For this review, take the finished solid that the model builds, in its own axes (mm). Coordinates: 2 decimals unless noted, no trailing zeros. Write each loop counter-clockwise with the first axis right and the second up, starting at its lowest first coordinate (ties: lowest second). Pieces come first, ordered by that corner, then holes. Notation, with made-up numbers: M -9,68 L 6,68 A9 cw 6,72 Z; hole C 17.5,64.25 d4. An arc over 180 degrees is marked long. Return JSON: item names as keys, results as strings.
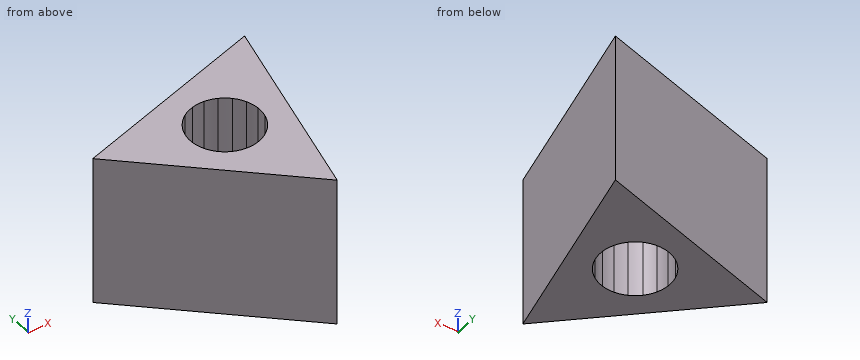
Autodesk Inventor part; units mm, degrees
ref_plane "Work Plane1" through (-2.6657, -0.4604, -13) normal (0, 0, -1) x (0, 1, 0)
ref_plane "YZ Plane" through (0, 0, 0) normal (1, 0, 0) x (0, 1, 0)
ref_plane "XZ Plane" through (0, 0, 0) normal (0, 1, 0) x (-1, 0, 0)
sketch "Sketch1" plane through (0, 0, 0) normal (0, 0, 1) x (1, 0, 0)
  line L0 (-1.6614, 3.5785) -> (-2.5268, 3.4417)
  line L1 (-2.0457, 4.3659) -> (-1.6614, 3.5785)
  line L2 (-1.1857, 4.1985) -> (-2.0457, 4.3659)
  line L3 (-1.2776, 5.0698) -> (-1.1857, 4.1985)
  line L4 (-0.5267, 4.6183) -> (-1.2776, 5.0698)
  line L5 (-0.315, 5.4685) -> (-0.5267, 4.6183)
  line L6 (-0.5267, 4.6183) -> (-0.315, 5.4685)
  arc A0 (-0.315, 5.4685) -> (-1.2776, 5.0698) centre (0.3343, 2.5396) ccw
  line L7 (-1.2776, 5.0698) -> (-0.5267, 4.6183)
  arc A1 (-1.2776, 5.0698) -> (-2.0457, 4.3659) centre (0.3343, 2.5396) ccw
  line L8 (-1.1857, 4.1985) -> (-1.2776, 5.0698)
  arc A2 (-1.2776, 5.0698) -> (-2.0457, 4.3659) centre (0.3343, 2.5396) ccw
  line L9 (-2.0457, 4.3659) -> (-1.1857, 4.1985)
  line L10 (-2.5268, 3.4417) -> (-1.6614, 3.5785)
  line L11 (-1.6614, 3.5785) -> (-2.0457, 4.3659)
  arc A3 (-2.0457, 4.3659) -> (-2.5268, 3.4417) centre (0.3343, 2.5396) ccw
  line L12 (0.2362, 4.7875) -> (0.7259, 5.5139)
  arc A4 (0.7259, 5.5139) -> (-0.315, 5.4685) centre (0.3343, 2.5396) ccw
  line L13 (-0.315, 5.4685) -> (0.2362, 4.7875)
  line L14 (1.0109, 4.6855) -> (1.7196, 5.2006)
  arc A5 (1.7196, 5.2006) -> (0.7259, 5.5139) centre (0.3343, 2.5396) ccw
  line L15 (0.7259, 5.5139) -> (1.0109, 4.6855)
  line L16 (1.7196, 5.2006) -> (1.7041, 4.3247)
  line L17 (1.7041, 4.3247) -> (2.5462, 4.5664)
  arc A6 (2.5462, 4.5664) -> (1.7196, 5.2006) centre (0.3343, 2.5396) ccw
  line L18 (2.5462, 4.5664) -> (2.232, 3.7485)
  line L19 (2.232, 3.7485) -> (3.106, 3.6877)
  arc A7 (3.106, 3.6877) -> (2.5462, 4.5664) centre (0.3343, 2.5396) ccw
  line L20 (3.106, 3.6877) -> (2.531, 3.0266)
  line L21 (2.531, 3.0266) -> (3.3315, 2.6705)
  arc A8 (3.3315, 2.6705) -> (3.106, 3.6877) centre (0.3343, 2.5396) ccw
  line L22 (-2.6628, 2.4087) -> (-2.632, 2.4258)
  line L23 (-2.632, 2.4258) -> (3.1702, 1.662)
  line L24 (3.1702, 1.662) -> (3.1955, 1.6375)
  arc A9 (3.1955, 1.6375) -> (3.3315, 2.6705) centre (0.3343, 2.5396) ccw
  line L25 (3.3315, 2.6705) -> (3.3007, 2.6534)
  line L26 (3.3007, 2.6534) -> (-2.5015, 3.4173)
  line L27 (-2.5015, 3.4173) -> (-2.5268, 3.4417)
  arc A10 (-2.5268, 3.4417) -> (-2.6628, 2.4087) centre (0.3343, 2.5396) ccw
  line L28 (3.1955, 1.6375) -> (2.3301, 1.5007)
  line L29 (2.3301, 1.5007) -> (2.7144, 0.7133)
  arc A11 (2.7144, 0.7133) -> (3.1955, 1.6375) centre (0.3343, 2.5396) ccw
  line L30 (2.7144, 0.7133) -> (1.8544, 0.8807)
  line L31 (1.8544, 0.8807) -> (1.9462, 0.0094)
  arc A12 (1.9462, 0.0094) -> (2.7144, 0.7133) centre (0.3343, 2.5396) ccw
  line L32 (1.1954, 0.4609) -> (0.9837, -0.3893)
  arc A13 (0.9837, -0.3893) -> (1.9462, 0.0094) centre (0.3343, 2.5396) ccw
  line L33 (1.9462, 0.0094) -> (1.1954, 0.4609)
  line L34 (0.4325, 0.2917) -> (-0.0572, -0.4347)
  arc A14 (-0.0572, -0.4347) -> (0.9837, -0.3893) centre (0.3343, 2.5396) ccw
  line L35 (0.9837, -0.3893) -> (0.4325, 0.2917)
  line L36 (-0.3422, 0.3937) -> (-1.0509, -0.1214)
  arc A15 (-1.0509, -0.1214) -> (-0.0572, -0.4347) centre (0.3343, 2.5396) ccw
  line L37 (-0.0572, -0.4347) -> (-0.3422, 0.3937)
  line L38 (-1.0354, 0.7546) -> (-1.8775, 0.5128)
  arc A16 (-1.8775, 0.5128) -> (-1.0509, -0.1214) centre (0.3343, 2.5396) ccw
  line L39 (-1.0509, -0.1214) -> (-1.0354, 0.7546)
  line L40 (-1.5633, 1.3307) -> (-2.4373, 1.3916)
  arc A17 (-2.4373, 1.3916) -> (-1.8775, 0.5128) centre (0.3343, 2.5396) ccw
  line L41 (-1.8775, 0.5128) -> (-1.5633, 1.3307)
  line L42 (-2.4373, 1.3916) -> (-1.8623, 2.0526)
  line L43 (-1.8623, 2.0526) -> (-2.6628, 2.4087)
  arc A18 (-2.6628, 2.4087) -> (-2.4373, 1.3916) centre (0.3343, 2.5396) ccw
  line L44 (2.9512, -7.1122) -> (-9.3328, 5.0993)
  line L45 (-9.3328, 5.0993) -> (7.3847, 9.6318)
  line L46 (7.3847, 9.6318) -> (2.9512, -7.1122)
  dimension "d0" = 17.321
ref_plane "Work Plane1" through (-2.6657, -0.4604, -13) normal (0, 0, -1) x (0, 1, 0)
extrude "Extrusion1" add sketch "Sketch1" against normal up to surface (13 mm away)
properties part number "HandlePotAttachmentGear"
1. We need section A-A (z = -5.75). State the section outline as (x, y) points (1 decimal), plus the area to 3 significant figures.
Checks:
{"outline": "M -9.3,5.1 L 3,-7.1 L 7.4,9.6 Z; hole M -2.7,2.4 A3 ccw -2.4,1.4 A3 ccw -1.9,0.5 A3 ccw -1.1,-0.1 A3 ccw -0.1,-0.4 A3 ccw 1,-0.4 A3 ccw 1.9,0 A3 ccw 2.7,0.7 A3 ccw 3.2,1.6 A3 ccw 3.3,2.7 A3 ccw 3.1,3.7 A3 ccw 2.5,4.6 A3 ccw 1.7,5.2 A3 ccw 0.7,5.5 A3 ccw -0.3,5.5 A3 ccw -1.3,5.1 A3 ccw -2,4.4 A3 ccw -2.5,3.4 A3 ccw Z", "area": "102 mm2"}
2. We need section D-D (y = 6.5). State the section outline as (x, z) points, plus the area to 3 significant figures.
Checks:
{"outline": "M -4.17,-13 L 6.56,-13 L 6.56,0 L -4.17,0 Z", "area": "139 mm2"}
3. Wall thickness on L1, parallel to Y at x = 1.5, z = -6.75; L2, parallel to Y at x = -8.25, z = -11; L3, parallel to Y at x = -1, z = -8: over which ranges is each line inside the solid? List them lowest first. Write a range as from..to.
Checks:
{"L1": "-5.67..-0.22, 5.3..8.04", "L2": "4.02..5.39", "L3": "-3.18..-0.15, 5.23..7.36"}
4. We need section C-C (x = -6.25). State the section outline as (y, z) points.
Checks:
{"outline": "M 2.03,-13 L 5.94,-13 L 5.94,0 L 2.03,0 Z"}
5. Clearance check with flat-ended pins moving along their axes: pin 1 Ø2 at (x, z) = (0, -2) entering from +Y; pin 2 Ø6 at (y, z) = (-4.5, -5.5) entering from +X; pin 3 Ø5 at (y, z) = (4.5, -7.5) entering from +X. State where each tip first meets the part, or that it passes through.
Checks:
{"pin 1": "y = 7.9", "pin 2": "x = 4.44", "pin 3": "x = 6.69"}
6. We need section B-B (y = 3). State the section outline as (x, z) points.
Checks:
{"outline": "M -7.22,-13 L -2.63,-13 L -2.63,0 L -7.22,0 Z; M 3.3,-13 L 5.63,-13 L 5.63,0 L 3.3,0 Z"}
